Could you check a few things on this model? Use its own coordinates, in mm. Give positions to 0.01 mm unless a question says otherwise; leave off trailing zeros. Write each loop counter-clockwise with the first axis right and the second up, starting at its lowest first coordinate (ties: lowest second). Pieces come first, ordered by that corner, then holes. Notation, with made-up numbers: M 8,75.5 L 46,75.5 A31 ccw 46,110.5 Z; hole C 86,75.25 d7. An arc over 180 degrees is marked long. Use one line per item in the form item = value.
from build123d import *

# Parameters (mm, degrees)
SKETCH1_R           = 4.1
BOSS_EXTRUDE1_DEPTH = 5


with BuildPart() as part:
    # Sketch1 → Boss-Extrude1 (new body)
    with BuildSketch(Plane(origin=(0, 0, 0), x_dir=(0, -1, 0), z_dir=(-1, 0, 0))):
        with BuildLine():
            Line((-13, 31.350852961), (-238, 161.254663529))
            ThreePointArc((-238, 161.254663529), (-262, 161.254663529), (-274, 140.470053838))
            Line((-274, 140.470053838), (-274, -23))
            ThreePointArc((-274, -23), (-273.707106781, -23.707106781), (-273, -24))
            Line((-273, -24), (-25, -24))
            ThreePointArc((-25, -24), (-8.029437252, -16.970562748), (-1, 0))
            Line((-1, 0), (-1, 10.56624327))
            ThreePointArc((-1, 10.56624327), (-4.215390309, 22.56624327), (-13, 31.350852961))
        make_face()
        with Locations((-255, 143.356805184)):
            Circle(SKETCH1_R, mode=Mode.SUBTRACT)
        with Locations((-255, 0)):
            Circle(SKETCH1_R, mode=Mode.SUBTRACT)
        with Locations((-28.5, 0)):
            Circle(SKETCH1_R, mode=Mode.SUBTRACT)
        with Locations((-87.5, 46.650635095)):
            Circle(SKETCH1_R, mode=Mode.SUBTRACT)
    extrude(amount=-BOSS_EXTRUDE1_DEPTH)


solid = part.part
1) I want a section at D-D, the plane y = 87.5. Please give me the cut outline in (x, z), plus the area to 3 significant figures.
Checked values:
outline = M 0,-24 L 5,-24 L 5,42.55 L 0,42.55 Z; M 0,50.75 L 5,50.75 L 5,74.36 L 0,74.36 Z
area = 451 mm2
2) Thinking about a two-plate mould opening in Z: for faces 1 (the cylindrical face through (2.46, 251.09, 144.59)), 2 (the cylindrical face through (2.46, 8.22, -17.16)), 3 (the flat face through (5, 170, 51)), which applies, released by +Z, released by -Z, zero draft, split by the parting line, or undercut?
Checked values:
face_1 = undercut
face_2 = released by -Z
face_3 = zero draft
3) I want a section at C-C, the plane y = 255. Please give me the cut outline in (x, z), plus the area to 3 significant figures.
Checked values:
outline = M 0,-24 L 5,-24 L 5,-4.1 L 0,-4.1 Z; M 0,4.1 L 5,4.1 L 5,139.26 L 0,139.26 Z; M 0,147.46 L 5,147.46 L 5,163.94 L 0,163.94 Z
area = 858 mm2
4) I want a section at B-B, the plane x = 0.75. Please give me the cut outline in (y, z).
Checked values:
outline = M 1,0 A24 ccw 25,-24 L 273,-24 A1 ccw 274,-23 L 274,140.47 A24 ccw 238,161.25 L 13,31.35 A24 ccw 1,10.57 Z; hole C 28.5,0 d8.2; hole C 87.5,46.65 d8.2; hole C 255,0 d8.2; hole C 255,143.36 d8.2
5) If I drill on L1, parallel to Z at x = 3.7, y = 255; L2, parallel to Z at x = 4.1, y = 248.5; L3, parallel to Z at x = 3.25, y = 87.5, over which ranges is the centre line in solid material (lowest first)?
Checked values:
L1 = -24 to -4.1, 4.1 to 139.26, 147.46 to 163.94
L2 = -24 to 164.42
L3 = -24 to 42.55, 50.75 to 74.36
6) I want a section at A-A, the plane y = 28.5. Please give me the cut outline in (x, z).
Checked values:
outline = M 0,-24 L 5,-24 L 5,-4.1 L 0,-4.1 Z; M 0,4.1 L 5,4.1 L 5,40.3 L 0,40.3 Z
7) For pin 1 Ø1 at (x, z) = (1, 24) entering from -Y; pin 2 Ø10.5 at (y, z) = (255, 0) entering from -X; pin 3 Ø1.5 at (x, y) = (2.5, 118.5) entering from +Z; pin 4 Ø3 at (x, y) = (4, 176.5) entering from +Z, each with a flat end and sliding along its axis, tell me the tip position at first contact or that it passes through.
Checked values:
pin_1 = 4.78
pin_2 = 0
pin_3 = 92.69
pin_4 = 126.61
